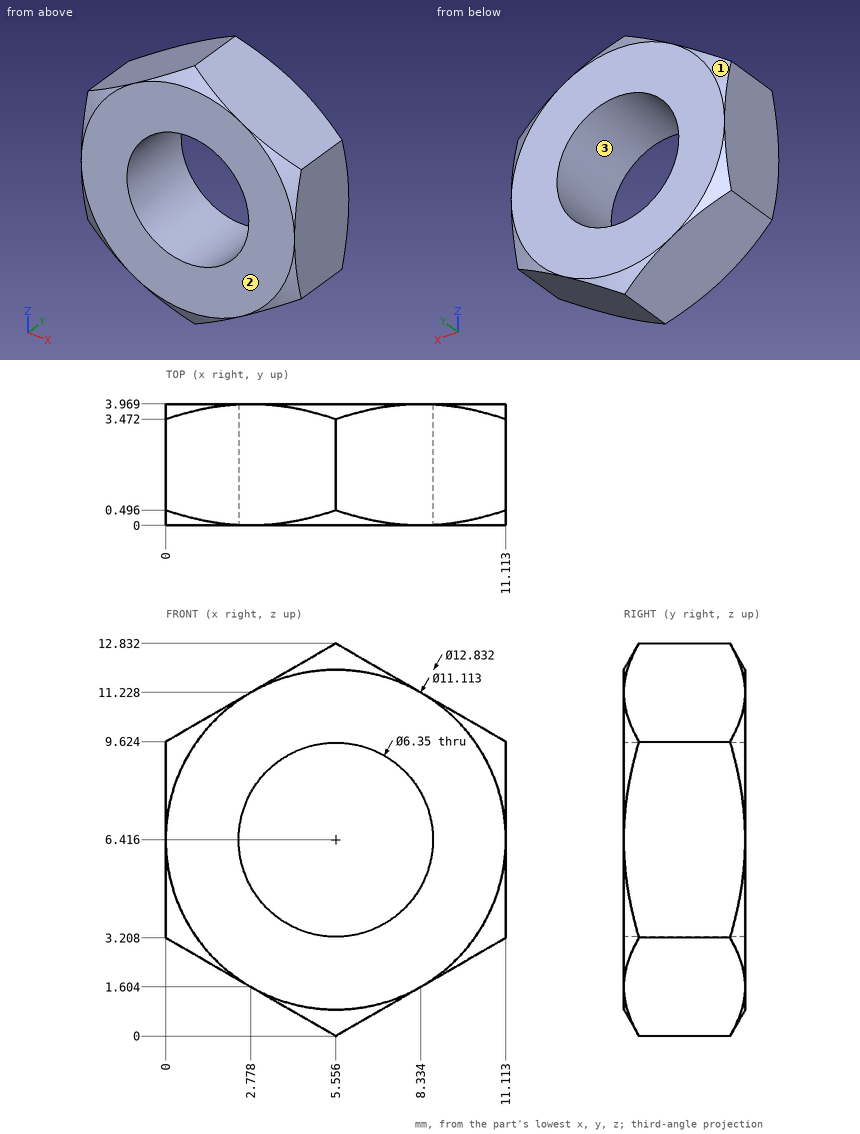
Here's the drawing with two shaded views (mm, measured from the low corner). I have some questions. Coordinates: 2 decimals unless noted, no trailing zeros. Use CSV: the item, a comma, the result in double quotes. Start each with the question number.
1. I'm going to push a flat-ended pin straight in: pin 1 (2 mm diameter, centred on x = 9.5, y = 2.5, fed in from -Z). Where does the tip first touch, or does it pass through?
2. Please list where these lines run through material, in increasing order: line 1 (X direction, y = 2.05, z = 9) (1 decimal); line 2 (Z direction, x = 3.5, y = 3.05) (1 decimal); line 3 (Z direction, x = 6.75, y = 0.65) (1 decimal). Write a range as from..to.
3. If we mould it in two halves opening along X, with no side actions, what happens to the marked faces 1, 2 and 3? For each: +X half, -X half, draft (parallel to the pull), parting line (faces both ways), or undercut.
Output:
1,pin 1,"stops at z = 1.7"
2,line 1,"x = 0..3.7, 7.4..11.1"
2,line 2,"z = 1.2..4, 8.8..11.6"
2,line 3,"z = 0.7..3.5, 9.4..12.1"
3,face 1,"-X half"
3,face 2,"draft"
3,face 3,"undercut"
